```python
from build123d import *

# Parameters (mm, degrees)
SKETCH1_W                 = 35
SKETCH1_H                 = 35
BOSS_EXTRUDE1_DEPTH       = 35
SKETCH2_R                 = 3.75
BOSS_EXTRUDE2_DEPTH       = 15
FILLET1_R                 = 1
F_2_0MM_DOWEL_HOLE1_D     = 2
F_2_0MM_DOWEL_HOLE1_DEPTH = 10
F_2_0MM_DOWEL_HOLE1_TIP   = 0.600860619


with BuildPart() as part:
    # Sketch1 → Boss-Extrude1 (new body)
    with BuildSketch(Plane(origin=(0, 0, 0), x_dir=(1, 0, 0), z_dir=(0, 1, 0))):
        Rectangle(SKETCH1_W, SKETCH1_H)
    extrude(amount=BOSS_EXTRUDE1_DEPTH)

    # Sketch2 → Boss-Extrude2 (add)
    with BuildSketch(Plane(origin=(0, 35, 0), x_dir=(1, 0, 0), z_dir=(0, 1, 0))):
        with Locations(Location((0, 0, 0), (0, 0, 270))):
            Circle(SKETCH2_R)
    extrude(amount=BOSS_EXTRUDE2_DEPTH)

    # Fillet1
    fillet1_edges = [part.edges().sort_by_distance(p)[0] for p in [
        (-17.5, 35, 0),
        (0, 35, 17.5),
        (0, 35, -3.75),
        (17.5, 35, 0),
        (0, 0, 17.5),
        (-17.5, 0, 0),
        (0, 0, -17.5),
        (17.5, 0, 0),
        (0, 35, -17.5),
        (17.5, 17.5, 17.5),
        (-17.5, 17.5, 17.5),
        (-17.5, 17.5, -17.5),
        (17.5, 17.5, -17.5),
    ]]
    fillet(fillet1_edges, radius=FILLET1_R)

    # Ø2.0mm Dowel Hole1
    with Locations(Plane(origin=(0, 35, 0), x_dir=(1, 0, 0), z_dir=(0, 1, 0))):
        with Locations((-15, 15), (15, 15), (15, -15), (-15, -15)):
            Hole(F_2_0MM_DOWEL_HOLE1_D / 2, depth=F_2_0MM_DOWEL_HOLE1_DEPTH)
            with Locations((0, 0, -(F_2_0MM_DOWEL_HOLE1_DEPTH + F_2_0MM_DOWEL_HOLE1_TIP / 2))):  # 118° drill point
                Cone(0, F_2_0MM_DOWEL_HOLE1_D / 2, F_2_0MM_DOWEL_HOLE1_TIP, mode=Mode.SUBTRACT)


solid = part.part
```
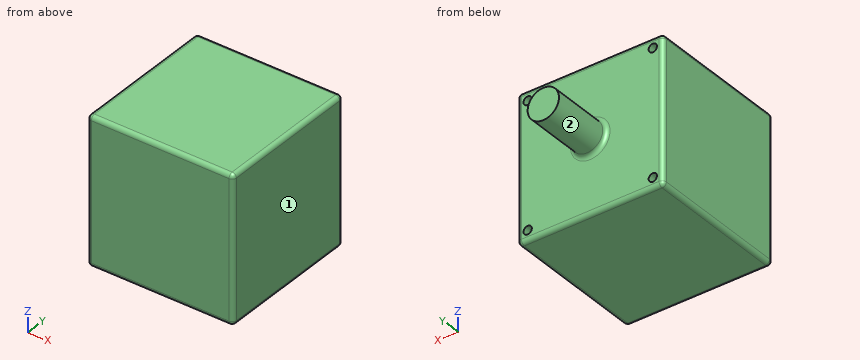
The listing builds one solid part. Answer for the finished solid, in the listing's coordinates (mm). Face numbers are marked on the shaded views. A direction names the side the tool comes from. Give positions to 0.01 mm unless a question says otherwise; leave off trailing zeros. Write each loop counter-clockwise with the first axis right and the second up, starting at its lowest first coordinate (ties: lowest second). Pieces come first, ordered by that corner, then holes. Notation, with made-up numbers: (-39, 30) -> (19, 30) arc R34 cw to (19, 64) -> close; hole circle Ø4 at (-17, -4). An arc over 180 degrees is marked (long way). Use one line per item in the form item = value.
1) Straight lines are drawn through the part: probe 1 along X at (y, z) = (29.75, -15); probe 2 along Y at (x, z) = (-11, -12.5). For each, find the intervals that lie inside material, in ascending order.
Result:
probe_1 = -17.5 to -16, -14 to 14, 16 to 17.5
probe_2 = 0 to 35
2) Section C-C on x = 0 is taken. Write down the section's boundary in (y, z), plus the area to 3 significant figures.
Result:
outline = (0, -16.5) arc R1 ccw to (1, -17.5) -> (34, -17.5) arc R1 ccw to (35, -16.5) -> (35, -4.75) arc R1 cw to (36, -3.75) -> (50, -3.75) -> (50, 3.75) -> (36, 3.75) arc R1 cw to (35, 4.75) -> (35, 16.5) arc R1 ccw to (34, 17.5) -> (1, 17.5) arc R1 ccw to (0, 16.5) -> close
area = 1,340 mm²
3) A tool of negligible diameter and unlimited length cuts with its end or side. For the marked faces 1 and 2, from which of +Z, -Z, +X, -X, +Y, -Y can it reach the whole face along a straight path? Write none if from no direction.
Result:
face_1 = +Z, -Z, +X, +Y, -Y
face_2 = +Y
4) Section A-A on z = 13 is taken. Write down the section's boundary in (x, y), plus the area to 3 significant figures.
Result:
outline = (-17.5, 1) arc R1 ccw to (-16.5, 0) -> (16.5, 0) arc R1 ccw to (17.5, 1) -> (17.5, 34) arc R1 ccw to (16.5, 35) -> (-16.5, 35) arc R1 ccw to (-17.5, 34) -> close
area = 1,220 mm²
5) Section D-D on z = 0 is taken. Write down the section's boundary in (x, y).
Result:
outline = (-17.5, 1) arc R1 ccw to (-16.5, 0) -> (16.5, 0) arc R1 ccw to (17.5, 1) -> (17.5, 34) arc R1 ccw to (16.5, 35) -> (4.75, 35) arc R1 cw to (3.75, 36) -> (3.75, 50) -> (-3.75, 50) -> (-3.75, 36) arc R1 cw to (-4.75, 35) -> (-16.5, 35) arc R1 ccw to (-17.5, 34) -> close
6) Each of these flat-tipped pins is pushed along its axis until it touches: P1, Ø12, axis at y = 43, z = -2.5, coming from the +X side; P2, Ø1.8, axis at x = 15, z = 15, coming from the +Y side; P3, Ø10, axis at x = 8, z = 4.5, coming from the +Y side; P4, Ø12, axis at x = -3.5, z = -7, coming from the +Y side. Where does it stop, or does it pass through?
Result:
P1 = 3.75
P2 = 24.94
P3 = 35.18
P4 = 50
7) Section B-B on x = -6 is taken. Write down the section's boundary in (y, z).
Result:
outline = (0, -16.5) arc R1 ccw to (1, -17.5) -> (34, -17.5) arc R1 ccw to (35, -16.5) -> (35, 16.5) arc R1 ccw to (34, 17.5) -> (1, 17.5) arc R1 ccw to (0, 16.5) -> close
